```python
from build123d import *

# Parameters (mm, degrees)
SKETCH1_W               = 406.4
SKETCH1_H               = 152.4
SKETCH1_W_2             = 401.32
SKETCH1_H_2             = 147.32
BOSS_EXTRUDE1_DEPTH     = 304.8
SKETCH2_W               = 406.4
SKETCH2_H               = 152.4
BOSS_EXTRUDE2_DEPTH     = 2.54
SKETCH3_W               = 12.7
SKETCH3_H               = 177.8
CUT_EXTRUDE1_DEPTH      = 1
CUT_EXTRUDE1_DEPTH_BACK = 407.4


with BuildPart() as part:
    # Sketch1 → Boss-Extrude1 (new body)
    with BuildSketch(Plane(origin=(0, 0, 0), x_dir=(1, 0, 0), z_dir=(0, 1, 0))):
        Rectangle(SKETCH1_W, SKETCH1_H)
        Rectangle(SKETCH1_W_2, SKETCH1_H_2, mode=Mode.SUBTRACT)
    extrude(amount=BOSS_EXTRUDE1_DEPTH)

    # Sketch2 → Boss-Extrude2 (add)
    with BuildSketch(Plane.XZ):
        Rectangle(SKETCH2_W, SKETCH2_H)
    extrude(amount=BOSS_EXTRUDE2_DEPTH)

    # Sketch3 → Cut-Extrude1 (cut, two sides)
    with BuildSketch(Plane.ZY.offset(203.2)) as cut_extrude1_sk:
        with Locations((44.45, 162.56)):
            Rectangle(SKETCH3_W, SKETCH3_H)
        with Locations((-31.75, 162.56)):
            Rectangle(SKETCH3_W, SKETCH3_H)
    extrude(amount=CUT_EXTRUDE1_DEPTH, mode=Mode.SUBTRACT)
    extrude(cut_extrude1_sk.sketch, amount=-CUT_EXTRUDE1_DEPTH_BACK, mode=Mode.SUBTRACT)


solid = part.part
```
Can you work these out from the model? Positions are in its coordinate system, mm. A direction names the side the tool comes from. Give positions to 0.01 mm unless a question says otherwise; leave off trailing zeros. Write each loop counter-clockwise with the first axis right and the second up, starting at its lowest first coordinate (ties: lowest second). Pieces come first, ordered by that corner, then holes. Notation, with made-up numbers: (-39, 63) - (-3, 63) arc R21 ccw to (-3, 75) - close; hole circle Ø5 at (30, -1). An arc over 180 degrees is marked (long way). Write item = value, one per line. Start each with the question number.
1. Imagine slicing it at C-C (z = 60.5). Please give me the cut outline in (x, y), and give its area (3 significant figures).
2. Imagine slicing it at D-D (x = -44). Please give me the cut outline in (y, z), and give its area (3 significant figures).
3. Imagine slicing it at B-B (y = 30.5). Please give me the cut outline in (x, z).
4. For pin 1 (5 mm diameter, centred on x = -7.5, z = 11, fed in from +Y), with a flat end and sliding along its axis, tell me the tip position at first contact or that it passes through.
5. On a 3-axis mill with a long thin cutter (end or side, diameter ignored), from which of +Z, -Z, +X, -X, +Y, -Y can I reach the whole of each face in a straight line? I mean faces 5 (the face through (-3, 150, -73.66)), 6 (the face through (203.2, 153, -1)). Say none if no direction works.
6. Thinking about a two-plate mould opening in X: for faces 1 (the face through (200.66, 150, 1)), 2 (the face through (-3, 153, -76.2)), 3 (the face through (-203.2, 153, -1)), 4 (the face through (-200.66, 150, 1)), which applies, released by +X, released by -X, zero draft, split by the parting line, or undercut?
7. Please list where these lines run through material, in increasing order: line 1 (Z direction, x = -30, y = 185); line 2 (X direction, y = 189.5, z = -41); line 3 (Y direction, x = -130.5, z = -57).
8. Imagine slicing it at A-A (y = 125). Please give me the cut outline in (x, z).
Worked answers:
q1.outline = (-203.2, -2.54) - (203.2, -2.54) - (203.2, 304.8) - (200.66, 304.8) - (200.66, 0) - (-200.66, 0) - (-200.66, 304.8) - (-203.2, 304.8) - close
q1.area = 2,580 mm2
q2.outline = (-2.54, -76.2) - (304.8, -76.2) - (304.8, -73.66) - (0, -73.66) - (0, 73.66) - (304.8, 73.66) - (304.8, 76.2) - (-2.54, 76.2) - close
q2.area = 1,940 mm2
q3.outline = (-203.2, -76.2) - (203.2, -76.2) - (203.2, 76.2) - (-203.2, 76.2) - close; hole (-200.66, -73.66) - (200.66, -73.66) - (200.66, 73.66) - (-200.66, 73.66) - close
q4.pin_1 = 0
q5.face_5 = +Y
q5.face_6 = +Z, -Z, +X, +Y, -Y
q6.face_1 = undercut
q6.face_2 = zero draft
q6.face_3 = released by -X
q6.face_4 = undercut
q7.line_1 = -76.2 to -73.66, 73.66 to 76.2
q7.line_2 = -203.2 to -200.66, 200.66 to 203.2
q7.line_3 = -2.54 to 0
q8.outline = (-203.2, -76.2) - (203.2, -76.2) - (203.2, -38.1) - (200.66, -38.1) - (200.66, -73.66) - (-200.66, -73.66) - (-200.66, -38.1) - (-203.2, -38.1) - close; (-203.2, -25.4) - (-200.66, -25.4) - (-200.66, 38.1) - (-203.2, 38.1) - close; (-203.2, 50.8) - (-200.66, 50.8) - (-200.66, 73.66) - (200.66, 73.66) - (200.66, 50.8) - (203.2, 50.8) - (203.2, 76.2) - (-203.2, 76.2) - close; (200.66, -25.4) - (203.2, -25.4) - (203.2, 38.1) - (200.66, 38.1) - close
